from build123d import *

# Parameters (mm, degrees)
F0_W     = 50
F0_H     = 75
F1_DEPTH = 2
F2_R     = 4.875
F3_DEPTH = 10
F5_DEPTH = 25


with BuildPart() as f1:
    # F0 (on Top) → F1 (new body)
    with BuildSketch(Plane.XY):
        Rectangle(F0_W, F0_H)
    extrude(amount=F1_DEPTH)

    # F2 (on face) → F3 (join)
    with BuildSketch(Plane.XY.offset(2)):
        Circle(F2_R)
    extrude(amount=F3_DEPTH)

    # F4 (on face) → F5 (cut)
    with BuildSketch(Plane.XY.offset(2)):
        with BuildLine():
            ThreePointArc((18.473266, -16.651813), (20.594587, -15.773133), (21.473266, -13.651813))
            Line((21.473266, -13.651813), (21.473266, -9.756987))
            ThreePointArc((21.473266, -9.756987), (20.594587, -7.635667), (18.473266, -6.756987))
            Line((18.473266, -6.756987), (-18.444779, -6.756987))
            ThreePointArc((-18.444779, -6.756987), (-20.566099, -7.635667), (-21.444779, -9.756987))
            Line((-21.444779, -9.756987), (-21.444779, -13.651813))
            ThreePointArc((-21.444779, -13.651813), (-20.566099, -15.773133), (-18.444779, -16.651813))
            Line((-18.444779, -16.651813), (18.473266, -16.651813))
        make_face()
        with BuildLine():
            Line((18.473266, 16.651813), (-18.444779, 16.651813))
            ThreePointArc((-18.444779, 16.651813), (-20.566099, 15.773133), (-21.444779, 13.651813))
            Line((-21.444779, 13.651813), (-21.444779, 9.756987))
            ThreePointArc((-21.444779, 9.756987), (-20.566099, 7.635667), (-18.444779, 6.756987))
            Line((-18.444779, 6.756987), (18.473266, 6.756987))
            ThreePointArc((18.473266, 6.756987), (20.594587, 7.635667), (21.473266, 9.756987))
            Line((21.473266, 9.756987), (21.473266, 13.651813))
            ThreePointArc((21.473266, 13.651813), (20.594587, 15.773133), (18.473266, 16.651813))
        make_face()
        with BuildLine():
            Line((18.473266, -18.756987), (-18.444779, -18.756987))
            ThreePointArc((-18.444779, -18.756987), (-20.566099, -19.635667), (-21.444779, -21.756987))
            Line((-21.444779, -21.756987), (-21.444779, -25.651813))
            ThreePointArc((-21.444779, -25.651813), (-20.566099, -27.773133), (-18.444779, -28.651813))
            Line((-18.444779, -28.651813), (18.473266, -28.651813))
            ThreePointArc((18.473266, -28.651813), (20.594587, -27.773133), (21.473266, -25.651813))
            Line((21.473266, -25.651813), (21.473266, -21.756987))
            ThreePointArc((21.473266, -21.756987), (20.594587, -19.635667), (18.473266, -18.756987))
        make_face()
        with BuildLine():
            Line((21.473266, 21.756987), (21.473266, 25.651813))
            ThreePointArc((21.473266, 25.651813), (20.594587, 27.773133), (18.473266, 28.651813))
            Line((18.473266, 28.651813), (-18.444779, 28.651813))
            ThreePointArc((-18.444779, 28.651813), (-20.566099, 27.773133), (-21.444779, 25.651813))
            Line((-21.444779, 25.651813), (-21.444779, 21.756987))
            ThreePointArc((-21.444779, 21.756987), (-20.566099, 19.635667), (-18.444779, 18.756987))
            Line((-18.444779, 18.756987), (18.473266, 18.756987))
            ThreePointArc((18.473266, 18.756987), (20.594587, 19.635667), (21.473266, 21.756987))
        make_face()
    extrude(amount=-F5_DEPTH, mode=Mode.SUBTRACT)


solid = f1.part
The model under review builds one solid part; all positions refer to its coordinate system, in mm. A direction names the side the tool comes from. Give positions to 0.01 mm unless a question says otherwise; leave off trailing zeros. Write each loop counter-clockwise with the first axis right and the second up, starting at its lowest first coordinate (ties: lowest second). Pieces come first, ordered by that corner, then holes.
1. For P1, Ø8, axis at x = 0.5, y = -14, coming from the +Z side, flat-tipped, find the tip position at first contact; note if it passes through.
2. Add section D-D, the plane y = 0. Write out the cut boundary in (x, z) (3 decimals).
3. Add section C-C, the plane z = 1. Count the separate pieces of the cut face and the enclosed holes in it, plus the area to 3 significant figures.
4. Wall thickness on L1, parallel to X at y = -8, z = 1.25; L2, parallel to Z at x = -3.5, y = 31; L3, parallel to X at y = 27.5, z = 1.75: over which ranges is each line inside the solid? List them lowest first.
5. Draft analysis for pull direction Y (two halves, no side actions). For faces 1 (the flat face through (25, -1, 1)), 2 (the cylindrical face through (-20.54, 27.8, 1.01)), 3 (the flat face through (0, 18.757, 1)), state which applies: +Y half, -Y half, draft (parallel to the pull), parting line (faces both ways), or undercut.
6. Add section B-B, the plane y = 24. Write out the cut boundary in (x, z).
7. Tool access review of faces 4 (the flat face through (-25, -1, 1)), 5 (the cylindrical face through (20.62, -19.66, 1.01)): name each direction out of +Z, -Z, +X, -X, +Y, -Y from which nothing blocks a thin tool from reaching the whole face with its end or side.
8. Add section A-A, the plane x = 0. Write out the cut boundary in (y, z) (3 decimals), plus the area to 3 significant figures.
Worked answers:
1. P1: stops at z = 2
2. outline: (-25, 0) - (25, 0) - (25, 2) - (4.875, 2) - (4.875, 12) - (-4.875, 12) - (-4.875, 2) - (-25, 2) - close
3. separate pieces: 1
3. enclosed holes: 4
3. area: 2,080 mm2
4. L1: x = -25 to -20.88, 20.9 to 25
4. L2: z = 0 to 2
4. L3: x = -25 to -20.81, 20.84 to 25
5. face 1: draft
5. face 2: undercut
5. face 3: undercut
6. outline: (-25, 0) - (-21.44, 0) - (-21.44, 2) - (-25, 2) - close; (21.47, 0) - (25, 0) - (25, 2) - (21.47, 2) - close
7. face 4: +Z, -Z, -X, +Y, -Y
7. face 5: +Z, -Z
8. outline: (-37.5, 0) - (-28.652, 0) - (-28.652, 2) - (-37.5, 2) - close; (-18.757, 0) - (-16.652, 0) - (-16.652, 2) - (-18.757, 2) - close; (-6.757, 0) - (6.757, 0) - (6.757, 2) - (4.875, 2) - (4.875, 12) - (-4.875, 12) - (-4.875, 2) - (-6.757, 2) - close; (16.652, 0) - (18.757, 0) - (18.757, 2) - (16.652, 2) - close; (28.652, 0) - (37.5, 0) - (37.5, 2) - (28.652, 2) - close
8. area: 168 mm2
